Print and shaded views of the part. All mm, measured from the part's lowest x, y and z. Round coordinates to 2 decimals unless told otherwise and drop trailing zeros. Write each loop counter-clockwise with the first axis right and the second up, starting at its lowest first coordinate (ties: lowest second). Pieces come first, ordered by that corner, then holes. Notation, with made-up numbers: (-20, 57.5) -> (11, 57.5) arc R16 cw to (11, 66.5) -> close; hole circle Ø3 at (54.25, 47.25). An arc over 180 degrees is marked (long way). Return JSON: item names as keys, results as strings. Group by question number.
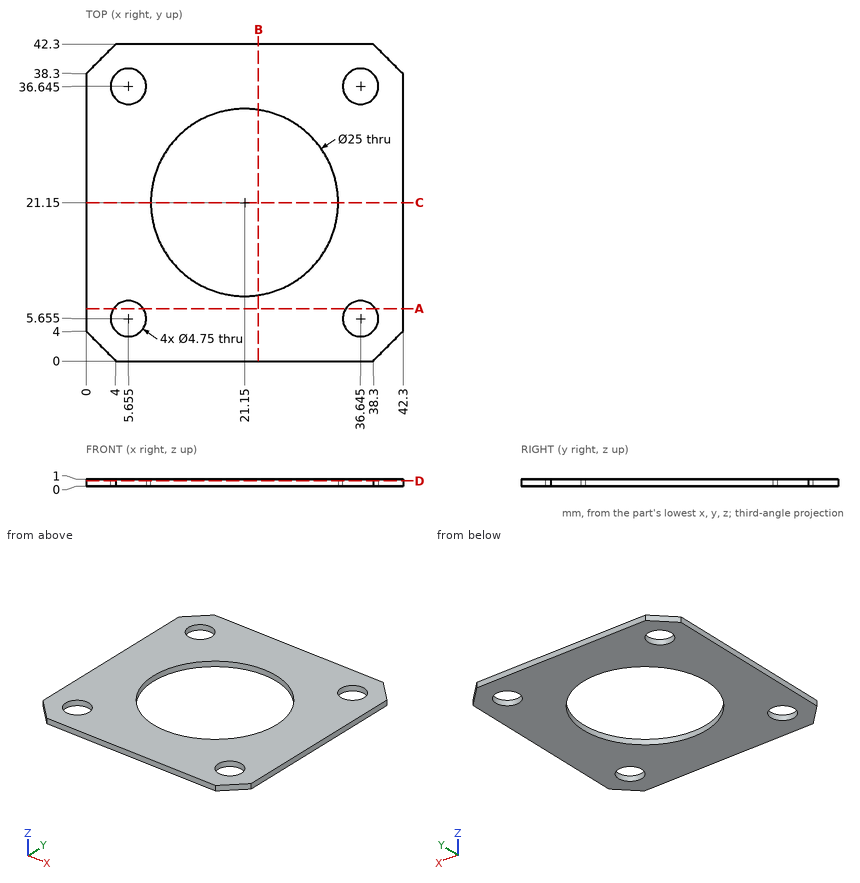
Item 1: Wall check: L1, parallel to Y at x = 36.5, z = 0.2; L2, parallel to Y at x = 21.15, z = 0.5. Give the ranges that are in metal, low to high.
Item 2: Cut at C-C (y = 21.15). Write the cut outline in (x, z), then the cut area to 3 significant figures.
Item 3: Cut at B-B (x = 23). Write the cut outline in (y, z), then the cut area to 3 significant figures.
Item 4: Cut at D-D (z = 0.75). Write the cut outline in (x, y) (3 decimals), then the cut area to 3 significant figures.
Item 5: Flat gauge pin, fed straight in: P1, Ø6, axis at x = 36.645, y = 5.655, coming from the -Z side. Where does the tip first touch, or does it go through?
Item 6: Cut at A-A (y = 7). Write the cut outline in (x, z).
Checks:
{
 "1": {"L1": "y = 0 to 3.28, 8.03 to 34.27, 39.02 to 42.3", "L2": "y = 0 to 8.65, 33.65 to 42.3"},
 "2": {"outline": "(0, 0) -> (8.65, 0) -> (8.65, 1) -> (0, 1) -> close; (33.65, 0) -> (42.3, 0) -> (42.3, 1) -> (33.65, 1) -> close", "area": "17.3 mm2"},
 "3": {"outline": "(0, 0) -> (8.79, 0) -> (8.79, 1) -> (0, 1) -> close; (33.51, 0) -> (42.3, 0) -> (42.3, 1) -> (33.51, 1) -> close", "area": "17.6 mm2"},
 "4": {"outline": "(0, 4) -> (4, 0) -> (38.3, 0) -> (42.3, 4) -> (42.3, 38.3) -> (38.3, 42.3) -> (4, 42.3) -> (0, 38.3) -> close; hole circle Ø4.75 at (5.655, 5.655); hole circle Ø4.75 at (5.655, 36.645); hole circle Ø25 at (21.15, 21.15); hole circle Ø4.75 at (36.645, 5.655); hole circle Ø4.75 at (36.645, 36.645)", "area": "1,200 mm2"},
 "5": {"P1": "stops at z = 0"},
 "6": {"outline": "(0, 0) -> (3.7, 0) -> (3.7, 1) -> (0, 1) -> close; (7.61, 0) -> (34.69, 0) -> (34.69, 1) -> (7.61, 1) -> close; (38.6, 0) -> (42.3, 0) -> (42.3, 1) -> (38.6, 1) -> close"}
}
